from build123d import *

# Parameters (mm, degrees)
EXTRUDE_1_DEPTH     = 5.5
CUT_EXTRUDE_START   = -2
CUT_EXTRUDE_1_DEPTH = 2
CUT_EXTRUDE_2_DEPTH = 2
EXTRUDE_2_DEPTH     = 5.5
SKETCH_5_R          = 2.75
EXTRUDE_3_DEPTH     = 3
SKETCH_6_R          = 1.5
EXTRUDE_4_DEPTH     = 20
SKETCH_7_R          = 1.5
EXTRUDE_5_DEPTH     = 7
EXTRUDE_START       = 3.5
SKETCH_8_R          = 1.5
EXTRUDE_6_DEPTH     = 3.5
EXTRUDE_7_DEPTH     = 3
EXTRUDE_8_DEPTH     = 7.5
EXTRUDE_9_DEPTH     = 6
SKETCH_12_R         = 2.369511938
SKETCH_12_R_2       = 1.4
CUT_EXTRUDE_3_DEPTH = 13.5


with BuildPart() as part:
    # Sketch 1 → Extrude 1 (new body)
    with BuildSketch(Plane(origin=(0, 0, 0), x_dir=(0, 0, -1), z_dir=(1, 0, 0))):
        with BuildLine():
            Line((-9.2, 0), (-0.630158831, -1.41612141))
            ThreePointArc((-0.630158831, -1.41612141), (0, -1.55), (0.630158831, -1.41612141))
            Line((0.630158831, -1.41612141), (9.2, 0))
            ThreePointArc((9.2, 0), (0, 9.2), (-9.2, 0))
        make_face()
    extrude(amount=EXTRUDE_1_DEPTH)

    # Sketch 2 → Cut-Extrude 1 (cut)
    with BuildSketch(Plane(origin=(5.5, 0, 0), x_dir=(0, 0, -1), z_dir=(1, 0, 0)).offset(CUT_EXTRUDE_START)):
        with BuildLine():
            Line((-7.994087674, 0.307509782), (-1.331520023, -0.79344466))
            ThreePointArc((-1.331520023, -0.79344466), (0, 1.55), (1.331520023, -0.79344466))
            Line((1.331520023, -0.79344466), (7.994087674, 0.307509782))
            ThreePointArc((7.994087674, 0.307509782), (0, 8), (-7.994087674, 0.307509782))
        make_face()
    extrude(amount=CUT_EXTRUDE_1_DEPTH, mode=Mode.SUBTRACT)

    # Sketch 3 → Cut-Extrude 2 (cut)
    with BuildSketch(Plane.ZY):
        with BuildLine():
            Line((-1.331520023, -0.79344466), (-7.994087674, 0.307509782))
            ThreePointArc((-7.994087674, 0.307509782), (0, 8), (7.994087674, 0.307509782))
            Line((7.994087674, 0.307509782), (1.331520023, -0.79344466))
            ThreePointArc((1.331520023, -0.79344466), (0, 1.55), (-1.331520023, -0.79344466))
        make_face()
    extrude(amount=-CUT_EXTRUDE_2_DEPTH, mode=Mode.SUBTRACT)

    # Sketch 4 → Extrude 2 (add)
    with BuildSketch(Plane.ZY):
        Polygon((0, 9.2), (-3.7, 9.2), (-3.7, 8.423182296), (3.7, 8.423182296), (3.7, 9.2), align=None)
    extrude(amount=-EXTRUDE_2_DEPTH)

    # Sketch 5 → Extrude 3 (add)
    with BuildSketch(Plane(origin=(0, 9.2, 0), x_dir=(1, 0, 0), z_dir=(0, 1, 0))):
        with Locations(Location((2.75, 0, 0), (0, 0, 180))):
            Circle(SKETCH_5_R)
    extrude(amount=EXTRUDE_3_DEPTH)

    # Fillet 1: read off the stored shape, not the designer's step
    # Fillet 1 outline → Fillet 1 (revolve, cut)
    with BuildSketch(Plane(origin=(2.75, 0, 0), x_dir=(1, 0, 0), z_dir=(0, 0, 1))):
        Polygon((2.75, 12.2), (2.05, 12.2), (2.75, 11.5), align=None)
    revolve(axis=Axis((2.75, 0, 0), (0, 1, 0)), mode=Mode.SUBTRACT)

    # Sketch 6 → Extrude 4 (add)
    with BuildSketch(Plane(origin=(0, 12.2, 0), x_dir=(1, 0, 0), z_dir=(0, 1, 0))):
        with Locations(Location((2.75, 0, 0), (0, 0, 270))):
            Circle(SKETCH_6_R)
    extrude(amount=EXTRUDE_4_DEPTH)

    # Sketch 7 → Extrude 5 (add)
    with BuildSketch(Plane.ZY):
        with Locations(Location((0, 0, 0), (0, 0, 180))):
            Circle(SKETCH_7_R)
    extrude(amount=EXTRUDE_5_DEPTH)

    # Sketch 8 → Extrude 6 (add)
    with BuildSketch(Plane(origin=(5.5, 0, 0), x_dir=(0, 0, -1), z_dir=(1, 0, 0)).offset(EXTRUDE_START)):
        Circle(SKETCH_8_R)
    extrude(amount=-EXTRUDE_6_DEPTH)

    # Sketch 9 → Extrude 7 (add)
    with BuildSketch(Plane(origin=(9, 0, 0), x_dir=(0, 0, -1), z_dir=(1, 0, 0))):
        Polygon((0, 1.2), (0.5, 1.2), (0.5, -1.2), (-0.5, -1.2), (-0.5, 1.2), align=None)
    extrude(amount=EXTRUDE_7_DEPTH)

    # Sketch 10 → Extrude 8 (add)
    with BuildSketch(Plane(origin=(4, 0, 0), x_dir=(0, 0, -1), z_dir=(1, 0, 0))):
        with BuildLine():
            Line((5.5, 0), (5, 0))
            Line((5, 0), (5, -0.694028023))
            Line((5, -0.694028023), (-2.5, -0.694028023))
            Line((-2.5, -0.694028023), (-2.5, 0))
            ThreePointArc((-2.5, 0), (-2.853553391, -0.146446609), (-3, -0.5))
            Line((-3, -0.5), (-3, -1.5))
            ThreePointArc((-3, -1.5), (-2.853553391, -1.853553391), (-2.5, -2))
            Line((-2.5, -2), (0, -2))
            Line((0, -2), (5.5, -2))
            ThreePointArc((5.5, -2), (5.853553391, -1.853553391), (6, -1.5))
            Line((6, -1.5), (6, -0.5))
            ThreePointArc((6, -0.5), (5.853553391, -0.146446609), (5.5, 0))
        make_face()
    extrude(amount=-EXTRUDE_8_DEPTH)

    # Sketch 11 → Extrude 9 (add)
    with BuildSketch(Plane.ZY.offset(-2)):
        with BuildLine():
            Line((-1.5, 0), (-1.5, 1.322875656))
            ThreePointArc((-1.5, 1.322875656), (0, 2), (1.5, 1.322875656))
            Line((1.5, 1.322875656), (1.599468005, -1.200709))
            ThreePointArc((1.599468005, -1.200709), (0.078769562, -1.998448237), (-1.5, -1.322875656))
            Line((-1.5, -1.322875656), (-1.5, 0))
        make_face()
    extrude(amount=EXTRUDE_9_DEPTH)

    # Sketch 12 → Cut-Extrude 3 (cut)
    with BuildSketch(Plane(origin=(0, 32.2, 0), x_dir=(1, 0, 0), z_dir=(0, 1, 0))):
        with Locations((2.75, 0)):
            Circle(SKETCH_12_R)
        with Locations(Location((2.75, 0, 0), (0, 0, 270))):
            Circle(SKETCH_12_R_2, mode=Mode.SUBTRACT)
    extrude(amount=-CUT_EXTRUDE_3_DEPTH, mode=Mode.SUBTRACT)


solid = part.part
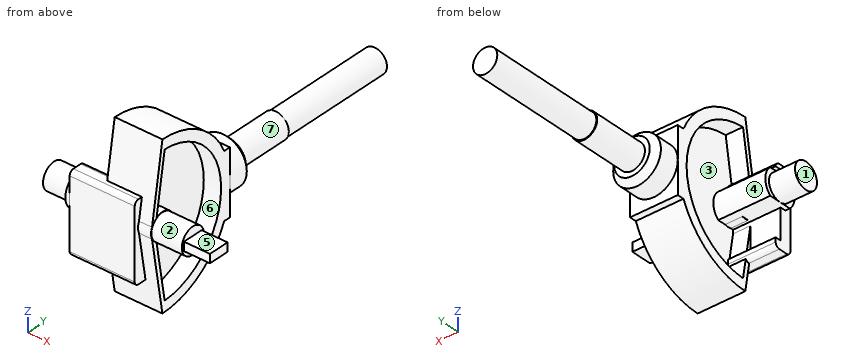
Could you check a few things on this model? Use its own coordinates, in mm. Face numbers are marked on the shaded views. A direction names the side the tool comes from. Round coordinates to 2 decimals unless told otherwise and drop trailing zeros. Write each loop counter-clockwise with the first axis right and the second up, starting at its lowest first coordinate (ties: lowest second). Pieces come first, ordered by that corner, then holes. Notation, with made-up numbers: (80.25, 75.25) - (111.25, 75.25) arc R19 ccw to (111.25, 83.25) - close; hole circle Ø4 at (-15.5, -32). An arc over 180 degrees is marked (long way). Use a Markdown table: item, result.
Q1. I want a section at A-A (x = 2.75). List the corners of the cut face in (y, z) for me, plus the area to 3 significant figures.
Output values:
| item | result |
|---|---|
| outline | (-2, -5.5) arc R0.5 ccw to (-1.5, -6) - (-0.53, -6) - (0, -9.2) arc R9.2 ccw to (8.42, -3.7) - (9.2, -3.7) - (9.2, -2.75) - (11.5, -2.75) - (12.2, -2.05) - (12.2, -1.5) - (18.7, -1.5) - (18.7, -1.4) - (32.2, -1.4) - (32.2, 1.4) - (18.7, 1.4) - (18.7, 1.5) - (12.2, 1.5) - (12.2, 2.05) - (11.5, 2.75) - (9.2, 2.75) - (9.2, 3.7) - (8.42, 3.7) arc R9.2 ccw to (0, 9.2) - (-1.02, 3) - (-1.5, 3) arc R0.5 ccw to (-2, 2.5) - close |
| area | 230 mm2 |
Q2. I want a section at C-C (x = -1). List the corners of the cut face in (y, z) for me, plus the area to 3 significant figures.
Output values:
| item | result |
|---|---|
| outline | (-2, -5.5) arc R0.5 ccw to (-1.5, -6) - (-0.5, -6) arc R0.5 ccw to (0, -5.5) - (0, -5) - (-0.69, -5) - (-0.69, -1.5) - (1.32, -1.5) arc R2 ccw to (1.32, 1.5) - (-0.69, 1.58) - (-0.69, 2.5) - (0, 2.5) arc R0.5 ccw to (-0.5, 3) - (-1.5, 3) arc R0.5 ccw to (-2, 2.5) - close |
| area | 20.1 mm2 |
Q3. Please list where these lines run through material, in increasing order: L1, parallel to Y at x = -2.75, z = -5.75; L2, parallel to Y at x = 4.5, z = 7.25; L3, parallel to Z at x = 5, y = 4.5.
Output values:
| item | result |
|---|---|
| L1 | -1.93 to -0.07 |
| L2 | -0.32 to 0.18, 3.38 to 5.66 |
| L3 | -8.02 to -6.61, 6.61 to 8.02 |
Q4. I want a section at B-B (y = 22.5). List the corners of the cut face in (x, z) for me, plus the area to 3 significant figures.
Output values:
| item | result |
|---|---|
| outline | circle Ø2.8 at (2.75, 0) |
| area | 6.16 mm2 |
Q5. I want a section at D-D (y = 13). List the corners of the cut face in (x, z) for me, plus the area to 3 significant figures.
Output values:
| item | result |
|---|---|
| outline | circle Ø3 at (2.75, 0) |
| area | 7.07 mm2 |
Q6. For pin 1 (0.6 mm diameter, centred on x = -1.5, y = -0.5, fed in from +Z); pin 2 (0.7 mm diameter, centred on x = 10, y = -0.5, fed in from -Z); pin 3 (6 mm diameter, centred on y = 25.5, z = -1.5, fed in from +X), each with a flat end and sliding along its axis, tell me the tip position at first contact or that it passes through.
Output values:
| item | result |
|---|---|
| pin 1 | z = 3 |
| pin 2 | z = -0.5 |
| pin 3 | x = 4.15 |
Q7. For the marked faces 4, 5, 6 and 7, which set-ups out of +Z, -Z, +X, -X, +Y, -Y let a thin tool reach every point of the face, with its end or its side?
Output values:
| item | result |
|---|---|
| face 4 | -X |
| face 5 | +Z, +X, +Y, -Y |
| face 6 | +X |
| face 7 | +Y |
Q8. Thinking about a two-plate mould opening in Y: for the marked faces 1, 2 and 3, which applies, released by +Y, released by -Y, zero draft, split by the parting line, or undercut?
Output values:
| item | result |
|---|---|
| face 1 | zero draft |
| face 2 | split by the parting line |
| face 3 | undercut |
